```python
from build123d import *

# Parameters (mm, degrees)
F0_R            = 140
F0_R_2          = 97
F1_DEPTH        = 112.5
F2_R            = 22.5
F3_DEPTH        = 32
F3_COPIES_COUNT = 3
F5_R            = 100
F7_R            = 28.1
F8_DEPTH        = 310
F9_R            = 50
F9_R_2          = 28.1
F10_DEPTH       = 25
F11_R           = 10.15
F12_DEPTH       = 15
F14_R           = 22.5
F14_R_2         = 97
F15_DEPTH       = 32


# Not quite as in the source:
# - a pattern or mirror of a feature is missing from the dataset's text; its kind, count and spacing are read off the source's solid
# - a feature names something its author has since deleted; it is built from what else it names


with BuildPart() as f1:
    # F0 (on Top) → F1 (new body, symmetric)
    with BuildSketch(Plane.XY):
        Circle(F0_R)
        Circle(F0_R_2, mode=Mode.SUBTRACT)
    extrude(amount=F1_DEPTH, both=True)

    # F2 (on face) → F3 (join)
    with BuildSketch(Plane(origin=(0, 0, -112.5), x_dir=(1, 0, 0), z_dir=(0, 0, -1))):
        with BuildLine():
            ThreePointArc((-44.1987298108, 176.5544456623), (-112.5, 194.8557158515), (-130.8012701892, 126.5544456623))
            Line((-130.8012701892, 126.5544456623), (-108.6847543423, 88.2475165291))
            ThreePointArc((-108.6847543423, 88.2475165291), (-70, 121.2435565298), (-22.0822139639, 138.2475165291))
            Line((-22.0822139639, 138.2475165291), (-44.1987298108, 176.5544456623))
        make_face()
        with Locations((-87.5, 151.5544456623)):
            Circle(F2_R, mode=Mode.SUBTRACT)
    f3 = extrude(amount=-F3_DEPTH)

    # F3_copies: F3 ×3 about axis
    f3_copies_axis = Axis((0, 0, 0), (0, 0, 1))
    for i in range(1, F3_COPIES_COUNT):
        add(f3.rotate(f3_copies_axis, i * 360 / F3_COPIES_COUNT))

    # F5 (on offset) → F6 (join, up to the next surface of F1)
    with BuildSketch(Plane.YZ.offset(-160)):
        Circle(F5_R)
    extrude(until=Until.NEXT)

    # F7 (on face) → F8 (cut)
    with BuildSketch(Plane(origin=(-160, 0, 0), x_dir=(0, -1, 0), z_dir=(-1, 0, 0))):
        Circle(F7_R)
    extrude(amount=-F8_DEPTH, mode=Mode.SUBTRACT)

    # F9 (on face) → F10 (cut)
    with BuildSketch(Plane(origin=(-160, 0, 0), x_dir=(0, -1, 0), z_dir=(-1, 0, 0))):
        Circle(F9_R)
        Circle(F9_R_2, mode=Mode.SUBTRACT)
    extrude(amount=-F10_DEPTH, mode=Mode.SUBTRACT)

    # F11 (on face) → F12 (cut)
    with BuildSketch(Plane(origin=(-160, 0, 0), x_dir=(0, -1, 0), z_dir=(-1, 0, 0))):
        with Locations((0, 79.0973976254)):
            Circle(F11_R)
        with Locations((-68.5003557169, -39.5486988127)):
            Circle(F11_R)
        with Locations((68.5003557169, -39.5486988127)):
            Circle(F11_R)
    extrude(amount=-F12_DEPTH, mode=Mode.SUBTRACT)

    # F14 (on face) → F15 (join)
    with BuildSketch(Plane.XY.offset(112.5)):
        with BuildLine():
            Line((-130.8012701892, 126.5544456623), (-108.6847543423, 88.2475165291))
            ThreePointArc((-108.6847543423, 88.2475165291), (-70, 121.2435565298), (-22.0822139639, 138.2475165291))
            Line((-22.0822139639, 138.2475165291), (-44.1987298108, 176.5544456623))
            ThreePointArc((-44.1987298108, 176.5544456623), (-112.5, 194.8557158515), (-130.8012701892, 126.5544456623))
        make_face()
        with Locations((-87.5, 151.5544456623)):
            Circle(F14_R, mode=Mode.SUBTRACT)
        with BuildLine():
            ThreePointArc((-22.0822139639, 138.2475165291), (-70, 121.2435565298), (-108.6847543423, 88.2475165291))
            ThreePointArc((-108.6847543423, 88.2475165291), (-140, 0), (-108.6847543423, -88.2475165291))
            ThreePointArc((-108.6847543423, -88.2475165291), (-70, -121.2435565298), (-22.0822139639, -138.2475165291))
            ThreePointArc((-22.0822139639, -138.2475165291), (70, -121.2435565298), (130.7669683062, -50))
            ThreePointArc((130.7669683062, -50), (137.6723929531, -25.4226713499), (140, 0))
            ThreePointArc((140, 0), (137.6723929531, 25.4226713499), (130.7669683062, 50))
            ThreePointArc((130.7669683062, 50), (70, 121.2435565298), (-22.0822139639, 138.2475165291))
        make_face()
        Circle(F14_R_2, mode=Mode.SUBTRACT)
        with BuildLine():
            ThreePointArc((-22.0822139639, -138.2475165291), (-70, -121.2435565298), (-108.6847543423, -88.2475165291))
            Line((-108.6847543423, -88.2475165291), (-130.8012701892, -126.5544456623))
            ThreePointArc((-130.8012701892, -126.5544456623), (-112.5, -194.8557158515), (-44.1987298108, -176.5544456623))
            Line((-44.1987298108, -176.5544456623), (-22.0822139639, -138.2475165291))
        make_face()
        with Locations((-87.5, -151.5544456623)):
            Circle(F14_R, mode=Mode.SUBTRACT)
        with BuildLine():
            Line((175, 50), (130.7669683062, 50))
            ThreePointArc((130.7669683062, 50), (137.6723929531, 25.4226713499), (140, 0))
            ThreePointArc((140, 0), (137.6723929531, -25.4226713499), (130.7669683062, -50))
            Line((130.7669683062, -50), (175, -50))
            ThreePointArc((175, -50), (225, 0), (175, 50))
        make_face()
        with Locations((175, 0)):
            Circle(F14_R, mode=Mode.SUBTRACT)
    extrude(amount=-F15_DEPTH)


solid = f1.part
```
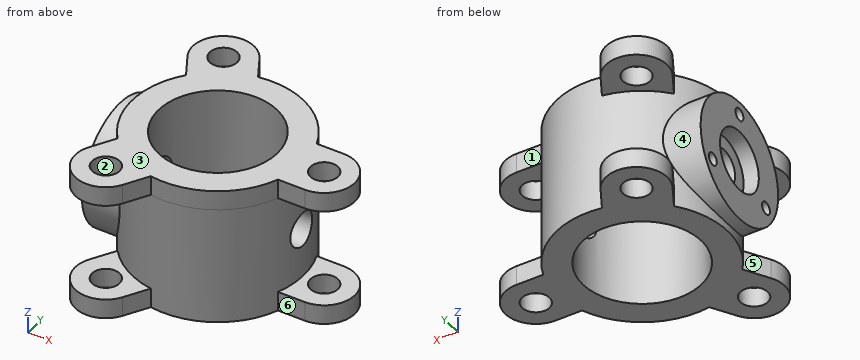
The listing builds one solid part. Answer for the finished solid, in the listing's coordinates (mm). Face numbers are marked on the shaded views. A direction names the side the tool comes from. Give positions to 0.01 mm unless a question says otherwise; leave off trailing zeros. Order: outer loops, then holes, each group sorted by start corner. A loop starts at its lowest first (then second) coordinate and runs counter-clockwise, first axis right, second up.
Item 1: For a pull along Y with two mould halves and no side action, classify the marked faces 1, 2 and 3 as pulls with the +Y half, pulls with the -Y half, needs draft (parallel to the pull), parting line crosses it, or undercut.
From the geometry:
face 1: pulls with the +Y half
face 2: undercut
face 3: needs draft
Item 2: The part is cut by section A-A, the plane x = 0. Give the vertices of the cut face in (y, z), and give its area (4 significant figures).
From the geometry:
outline: (-140, -112.5) - (-97, -112.5) - (-97, 112.5) - (-140, 112.5) - close; (97, -112.5) - (140, -112.5) - (140, 112.5) - (97, 112.5) - close
area: 19,350 mm2
Item 3: Given pin 1 Ø2 at (x, z) = (-52.5, -13.5) entering from -Y; pin 2 Ø9.5 at (x, z) = (144, 92) entering from +Y; pin 3 Ø10 at (y, z) = (-90.5, 66) entering from +X, each flat-ended and moving along its own axis, determine where each tip first touches the part or whether it passes through.
From the geometry:
pin 1: stops at y = -130.18
pin 2: stops at y = 50
pin 3: stops at x = 110.86
Item 4: The part is cut by section D-D, the plane x = -87.5. Count the separate pieces of the cut face and the enclosed holes in it, and give its area (3 significant figures).
From the geometry:
separate pieces: 6
enclosed holes: 0
area: 36,400 mm2
Item 5: Find the intervals of material crossed by probe 1 along Z at (x, y) = (159.5, 22); probe 2 along Y at (x, z) = (-87.5, -99.5); probe 3 along Y at (x, z) = (175, 101.5), in increasing order.
From the geometry:
probe 1: z = -112.5 to -80.5, 80.5 to 112.5
probe 2: y = -201.55 to -174.05, -129.05 to -41.87, 41.87 to 129.05, 174.05 to 201.55
probe 3: y = -50 to -22.5, 22.5 to 50
Item 6: Which of the six approach directions +Z, -Z, +X, -X, +Y, -Y give full straight-line access (tool end or side, diameter ignored) to the marked faces 4, 5 and 6?
From the geometry:
face 4: -X
face 5: -Z, -X
face 6: +Z, -Z, +X, -Y
Item 7: The part is cut by section B-B, the plane z = -10. Give the vertices of the cut face in (x, y).
From the geometry:
outline: (-160, -99.5) - (-98.49, -99.5) arc R140 ccw to (137.52, -26.26) - (93.38, -26.26) arc R97 cw to (-93.38, -26.26) - (-135, -26.26) - (-135, -48.99) - (-160, -48.99) - close; (-160, 48.99) - (-135, 48.99) - (-135, 26.26) - (-93.38, 26.26) arc R97 cw to (93.38, 26.26) - (137.52, 26.26) arc R140 ccw to (-98.49, 99.5) - (-160, 99.5) - close
Item 8: The part is cut by section C-C, the plane y = -160.5. Give the vertices of the cut face in (x, z).
From the geometry:
outline: (-136.69, -112.5) - (-108.15, -112.5) - (-108.15, -80.5) - (-136.69, -80.5) - close; (-136.69, 80.5) - (-108.15, 80.5) - (-108.15, 112.5) - (-136.69, 112.5) - close; (-66.85, -112.5) - (-34.93, -112.5) - (-34.93, -80.5) - (-66.85, -80.5) - close; (-66.85, 80.5) - (-34.93, 80.5) - (-34.93, 112.5) - (-66.85, 112.5) - close
